from build123d import *

# Parameters (mm, degrees)
SKETCH1_W                       = 9.13
SKETCH1_H                       = 0.3
BOSS_EXTRUDE1_DEPTH             = 11.42
BOSS_EXTRUDE3_DEPTH             = 0.3
BOSS_EXTRUDE4_DEPTH             = 0.3
FILLET2_R                       = 0.3
FILLET3_R                       = 0.6
BOSS_EXTRUDE5_REACH             = 14.701
BOSS_EXTRUDE5_DIRECTION_2_REACH = 14.701
FILLET4_R                       = 0.595


with BuildPart() as part:
    # Sketch1 → Boss-Extrude1 (new body)
    with BuildSketch(Plane(origin=(0, 0, 0), x_dir=(1, 0, 0), z_dir=(0, 1, 0))):
        Rectangle(SKETCH1_W, SKETCH1_H)
    extrude(amount=BOSS_EXTRUDE1_DEPTH)

    # Sketch3 → Boss-Extrude3 (add)
    with BuildSketch(Plane(origin=(0, 0, -0.15), x_dir=(-1, 0, 0), z_dir=(0, 0, -1))):
        with BuildLine():
            Line((-0.57, 0), (0.57, 0))
            Line((0.57, 0), (0.57, -1.6))
            Line((0.57, -1.6), (0.33, -2.770784784))
            ThreePointArc((0.33, -2.770784784), (0, -3.04), (-0.33, -2.770784784))
            Line((-0.33, -2.770784784), (-0.57, -1.6))
            Line((-0.57, -1.6), (-0.57, 0))
        make_face()
    extrude(amount=-BOSS_EXTRUDE3_DEPTH)

    # Sketch4 → Boss-Extrude4 (add)
    with BuildSketch(Plane(origin=(4.565, 0, 0), x_dir=(0, 0, -1), z_dir=(1, 0, 0))):
        with BuildLine():
            Line((-0.15, 11.42), (-0.15, 0))
            Line((-0.15, 0), (-1.425, 0))
            Line((-1.425, 0), (-1.425, 0.4))
            ThreePointArc((-1.425, 0.4), (-1.925, 0.9), (-2.425, 0.4))
            Line((-2.425, 0.4), (-2.425, 0))
            Line((-2.425, 0), (-3.615, 0))
            Line((-3.615, 0), (-3.615, 0.4))
            ThreePointArc((-3.615, 0.4), (-4.115, 0.9), (-4.615, 0.4))
            Line((-4.615, 0.4), (-4.615, 0))
            Line((-4.615, 0), (-6.19, 0))
            Line((-6.19, 0), (-6.19, 0.9))
            Line((-6.19, 0.9), (-2.4, 10.767226789))
            ThreePointArc((-2.4, 10.767226789), (-2.026327352, 11.241078061), (-1.45, 11.42))
            Line((-1.45, 11.42), (-0.15, 11.42))
        make_face()
    boss_extrude4 = extrude(amount=-BOSS_EXTRUDE4_DEPTH)

    # Fillet2
    fillet2_edges = [part.edges().sort_by_distance(p)[0] for p in [
        (4.265, 5.71, 0.15),
    ]]
    fillet(fillet2_edges, radius=FILLET2_R)

    # Fillet3
    fillet3_edges = [part.edges().sort_by_distance(p)[0] for p in [
        (4.565, 5.71, -0.15),
    ]]
    fillet(fillet3_edges, radius=FILLET3_R)

    # Boss-Extrude5: up to this face of the body (flat: up to its plane)
    boss_extrude5_end = Plane(part.part.faces().sort_by_distance((4.415, 0.2, 2.425))[0])
    # Sketch5 → Boss-Extrude5 (add, up to the picked face)
    with BuildSketch(Plane(origin=(0, 0, 3.02), x_dir=(-1, 0, 0), z_dir=(0, 0, -1)), mode=Mode.PRIVATE) as boss_extrude5_sk1:
        with BuildLine():
            Line((-4.565, 0), (-4.265, 0))
            Line((-4.265, 0), (-4.265, -0.734365081))
            ThreePointArc((-4.265, -0.734365081), (-4.31067228, -0.963975141), (-4.440735931, -1.15862915))
            Line((-4.440735931, -1.15862915), (-4.833553391, -1.551446609))
            ThreePointArc((-4.833553391, -1.551446609), (-4.966005966, -1.787534255), (-4.95599841, -2.058053958))
            Line((-4.95599841, -2.058053958), (-4.422200477, -3.718167625))
            Line((-4.422200477, -3.718167625), (-4.707799523, -3.81))
            Line((-4.707799523, -3.81), (-5.241597456, -2.149886332))
            ThreePointArc((-5.241597456, -2.149886332), (-5.257609545, -1.717054807), (-5.045685425, -1.339314575))
            Line((-5.045685425, -1.339314575), (-4.652867966, -0.946497116))
            ThreePointArc((-4.652867966, -0.946497116), (-4.58783614, -0.849170111), (-4.565, -0.734365081))
            Line((-4.565, -0.734365081), (-4.565, 0))
        make_face()
    boss_extrude5_tool1 = split(extrude(boss_extrude5_sk1.sketch, amount=BOSS_EXTRUDE5_REACH, mode=Mode.PRIVATE), bisect_by=boss_extrude5_end, keep=Keep.BOTH, mode=Mode.PRIVATE)
    boss_extrude5 = boss_extrude5_tool1.solids().sort_by(Axis((4.415, -0.039429, 3.02), (0, 0, -1)))[0]
    add(boss_extrude5)

    # Boss-Extrude5 direction 2: up to this face of the body (flat: up to its plane)
    boss_extrude5_direction_2_end = Plane(part.part.faces().sort_by_distance((4.415, 0.2, 3.615))[0])
    # Sketch5 → Boss-Extrude5 direction 2 (add, up to the picked face)
    with BuildSketch(Plane(origin=(0, 0, 3.02), x_dir=(-1, 0, 0), z_dir=(0, 0, -1)), mode=Mode.PRIVATE) as boss_extrude5_direction_2_sk1:
        with BuildLine():
            Line((-4.565, 0), (-4.265, 0))
            Line((-4.265, 0), (-4.265, -0.734365081))
            ThreePointArc((-4.265, -0.734365081), (-4.31067228, -0.963975141), (-4.440735931, -1.15862915))
            Line((-4.440735931, -1.15862915), (-4.833553391, -1.551446609))
            ThreePointArc((-4.833553391, -1.551446609), (-4.966005966, -1.787534255), (-4.95599841, -2.058053958))
            Line((-4.95599841, -2.058053958), (-4.422200477, -3.718167625))
            Line((-4.422200477, -3.718167625), (-4.707799523, -3.81))
            Line((-4.707799523, -3.81), (-5.241597456, -2.149886332))
            ThreePointArc((-5.241597456, -2.149886332), (-5.257609545, -1.717054807), (-5.045685425, -1.339314575))
            Line((-5.045685425, -1.339314575), (-4.652867966, -0.946497116))
            ThreePointArc((-4.652867966, -0.946497116), (-4.58783614, -0.849170111), (-4.565, -0.734365081))
            Line((-4.565, -0.734365081), (-4.565, 0))
        make_face()
    boss_extrude5_direction_2_tool1 = split(extrude(boss_extrude5_direction_2_sk1.sketch, amount=-BOSS_EXTRUDE5_DIRECTION_2_REACH, mode=Mode.PRIVATE), bisect_by=boss_extrude5_direction_2_end, keep=Keep.BOTH, mode=Mode.PRIVATE)
    boss_extrude5_direction_2 = boss_extrude5_direction_2_tool1.solids().sort_by(Axis((4.415, -0.039429, 3.02), (0, 0, 1)))[0]
    add(boss_extrude5_direction_2)

    # Fillet4
    fillet4_edges = [part.edges().sort_by_distance(p)[0] for p in [
        (4.565, -3.764083813, 2.425),
        (4.565, -3.764083813, 3.615),
    ]]
    fillet(fillet4_edges, radius=FILLET4_R - 0.0001)  # a hair under: the kernel refuses the full size

    # Mirror1: Boss-Extrude4, Boss-Extrude5, Boss-Extrude5 direction 2 across plane
    add(boss_extrude4.mirror(Plane(origin=(0, 0, 0), x_dir=(0, 0, 1), z_dir=(1, 0, 0))))
    add(boss_extrude5.mirror(Plane(origin=(0, 0, 0), x_dir=(0, 0, 1), z_dir=(1, 0, 0))))
    add(boss_extrude5_direction_2.mirror(Plane(origin=(0, 0, 0), x_dir=(0, 0, 1), z_dir=(1, 0, 0))))

    # Sketch7 → Revolve2 (revolve)
    with BuildSketch(Plane(origin=(0, 0, 0), x_dir=(0, 0, -1), z_dir=(1, 0, 0)), mode=Mode.PRIVATE) as revolve2_sk:
        with BuildLine():
            Line((0.15, 9.21), (0.436483674, 9.474099927))
            ThreePointArc((0.436483674, 9.474099927), (0.53, 9.6875), (0.436483674, 9.900900073))
            Line((0.436483674, 9.900900073), (0.15, 10.165))
            Line((0.15, 10.165), (0.15, 9.21))
        make_face()
    revolve(revolve2_sk.sketch.rotate(Axis((0, 6.99, -0.15), (0, 0, -1)), 90), axis=Axis((0, 6.99, -0.15), (0, 0, -1)))


solid = part.part
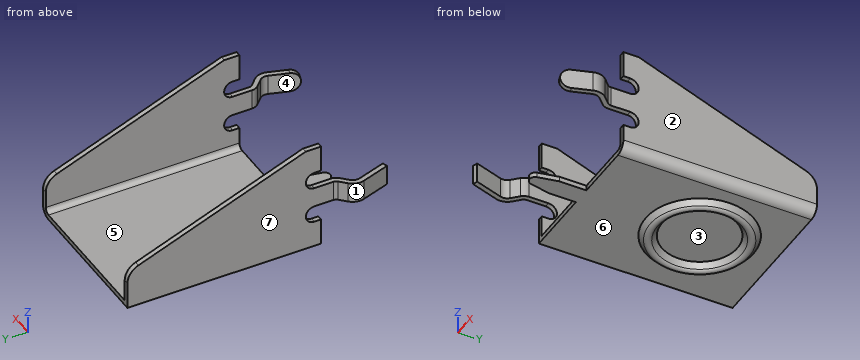
For this review, take the finished solid that the model builds, in its own axes (mm). Face numbers are marked on the shaded views. A direction names the side the tool comes from. Round coordinates to 2 decimals unless told otherwise and drop trailing zeros. Write each loop counter-clockwise with the first axis right and the second up, starting at its lowest first coordinate (ties: lowest second). Pieces come first, ordered by that corner, then holes. Notation, with made-up numbers: (-13.75, 56) -> (36.25, 56) arc R25 cw to (36.25, 77) -> close; hole circle Ø7 at (2.25, -33.75). An arc over 180 degrees is marked (long way). Put each result on its own line as item: value.
Q1. To check wall thickness, follow L1, parallel to X at y = 8.75, z = 1 (3 decimals); L2, parallel to Y at x = -2, z = 0; L3, parallel to Z at x = 3.5, y = 9. State the ranges of each line that lie inside material, in increasing order. Write a range as [from, to].
Determined:
L1: x = [-4.565, -4.265], [4.265, 4.565]
L2: y = [0, 11.42]
L3: z = [-0.15, 0.15]
Q2. Consider section A-A on y = -0.5. State the section outline as (x, z) points (3 decimals).
Determined:
outline: (-4.565, 2.425) -> (-4.265, 2.425) -> (-4.265, 3.615) -> (-4.565, 3.615) -> close; (-0.57, -0.15) -> (0.57, -0.15) -> (0.57, 0.15) -> (-0.57, 0.15) -> close; (4.265, 2.425) -> (4.565, 2.425) -> (4.565, 3.615) -> (4.265, 3.615) -> close
Q3. The part is to be moulded in two halves that separate along X. For the marked faces 1, 2 and 3, say which applies: released by +X, released by -X, zero draft, split by the parting line, or undercut.
Determined:
face 1: released by -X
face 2: released by +X
face 3: undercut
Q4. Machinability: for the marked faces 4, 5, 6 and 7, which of the approach directions +Z, -Z, +X, -X, +Y, -Y give a long, thin tool a straight path to every point of the face, cutting with its end or side? Answer none if there is none.
Determined:
face 4: +Z, -Z
face 5: +Z, +Y, -Y
face 6: -Z
face 7: +Z, -Z, -X, +Y
Q5. Consider section D-D on y = 1.75. State the section outline as (x, z) points (3 decimals), and give its area (3 significant figures).
Determined:
outline: (-4.565, -0.15) -> (3.965, -0.15) arc R0.6 ccw to (4.565, 0.45) -> (4.565, 5.864) -> (4.265, 5.864) -> (4.265, 0.45) arc R0.3 cw to (3.965, 0.15) -> (-4.265, 0.15) -> (-4.265, 5.864) -> (-4.565, 5.864) -> close
area: 6.11 mm^2
Q6. Clearance check with flat-ended pins moving along their axes: pin 1 Ø1.3 at (x, z) = (-2, 0.5) entering from -Y; pin 2 Ø2.5 at (x, y) = (-1, 7.5) entering from +Z; pin 3 Ø3 at (y, z) = (5, 2.5) entering from +X (3 decimals). State where each tip first meets the part, or that it passes through.
Determined:
pin 1: stops at y = 0
pin 2: stops at z = 0.15
pin 3: stops at x = 4.565
